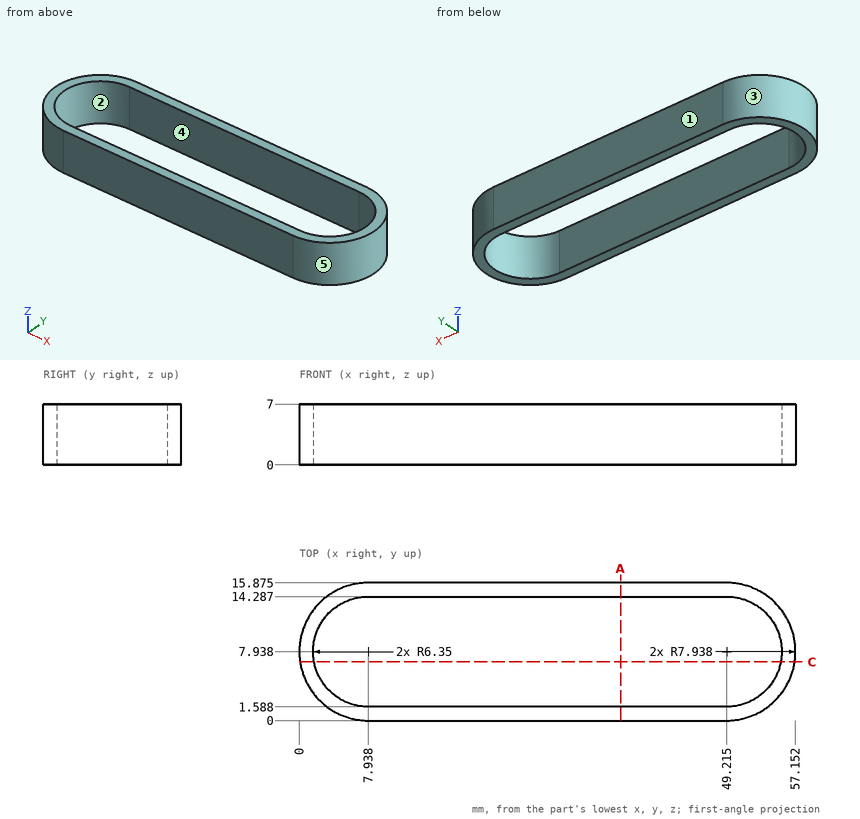
Job drawing, mm, ordinate dimensions from the low corner. One solid piece. A direction names the side the tool comes from. Round coordinates to 2 decimals unless told otherwise and drop trailing zeros. Order: outer loops, then holes, each group sorted by start corner. A loop starts at its lowest first (then second) coordinate and runs counter-clockwise, first axis right, second up. Notation, with made-up numbers: (-20, -10.75) -> (30, -10.75) arc R33 ccw to (30, 24.25) -> close; hole circle Ø5 at (73.5, -25.75). An arc over 180 degrees is marked (long way). Answer in a Markdown table with one row per item.
1) Which spindle directions (+Z, -Z, +X, -X, +Y, -Y) get a long thin tool onto all of the face, cutting with end or side? Do the marked faces 4 and 5. Say none if no direction does.
Values:
| item | result |
|---|---|
| face 4 | +Z, -Z |
| face 5 | +Z, -Z, +X |
2) Band-saw the part on C-C on y = 6.75. Give the cut face in (x, z).
Values:
| item | result |
|---|---|
| outline | (0.09, 0) -> (1.7, 0) -> (1.7, 7) -> (0.09, 7) -> close; (55.45, 0) -> (57.06, 0) -> (57.06, 7) -> (55.45, 7) -> close |
3) Pin check, flat tips, straight feed: P1, Ø3, axis at y = 4.5, z = 3, coming from the +X side; P2, Ø1, axis at y = 4.5, z = 3, coming from the +X side; P3, Ø1, axis at x = 33.5, y = 13, coming from the +Z side; P4, Ø1, axis at y = 3.5, z = 4, coming from the -X side (1 decimal). Stop position of each tip, or through.
Values:
| item | result |
|---|---|
| P1 | x = 56.91 |
| P2 | x = 56.59 |
| P3 | through |
| P4 | x = 1 |
4) Mould opens along X. For the marked faces 1, 2 and 3 say: released by +X, released by -X, zero draft, split by the parting line, or undercut.
Values:
| item | result |
|---|---|
| face 1 | zero draft |
| face 2 | undercut |
| face 3 | released by -X |
5) Wall check: L1, parallel to Y at x = 25, z = 0.75 (1 decimal); L2, parallel to X at y = 8, z = 5 (1 decimal); L3, parallel to X at y = 7.75, z = 3. Give the ranges that are in metal, low to high.
Values:
| item | result |
|---|---|
| L1 | 0 to 1.6, 14.3 to 15.9 |
| L2 | 0 to 1.6, 55.6 to 57.2 |
| L3 | 0 to 1.59, 55.56 to 57.15 |
6) Band-saw the part on A-A on x = 37. Give the cut face in (y, z) (1 decimal).
Values:
| item | result |
|---|---|
| outline | (0, 0) -> (1.6, 0) -> (1.6, 7) -> (0, 7) -> close; (14.3, 0) -> (15.9, 0) -> (15.9, 7) -> (14.3, 7) -> close |
